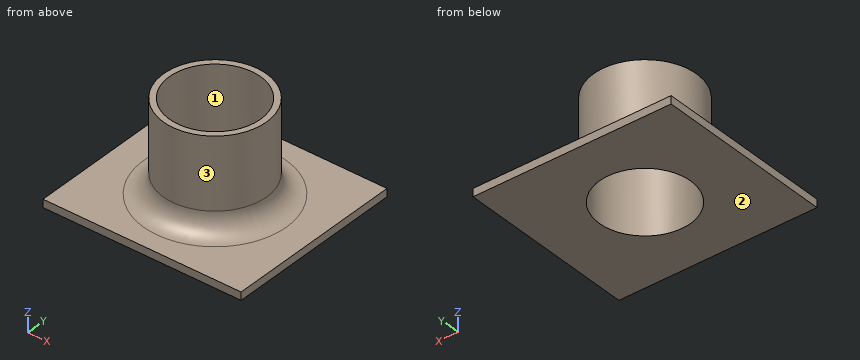
```python
from build123d import *

# Parameters (mm, degrees)
F1_W      = 50
F1_H      = 45.323998
F2_DEPTH  = 2
F0_R      = 13
F0_R_2    = 11.5
F3_DEPTH  = 25
F3_FACE_R = 11.5
F4_DEPTH  = 25
F5_R      = 5


with BuildPart() as f2:
    # F1 (on Top) → F2 (new body)
    with BuildSketch(Plane.XY):
        Rectangle(F1_W, F1_H)
    extrude(amount=F2_DEPTH)

    # F0 (on Top) → F3 (join)
    with BuildSketch(Plane.XY):
        Circle(F0_R)
        Circle(F0_R_2, mode=Mode.SUBTRACT)
    extrude(amount=F3_DEPTH)

    # F3_face (on face) → F4 (cut)
    with BuildSketch(Plane.XY.offset(2)):
        Circle(F3_FACE_R)
    extrude(amount=-F4_DEPTH, mode=Mode.SUBTRACT)

    # F5
    f5_edges = [f2.edges().sort_by_distance(p)[0] for p in [
        (-13, 0, 2),
    ]]
    fillet(f5_edges, radius=F5_R)


solid = f2.part
```
Can you work these out from the model? Positions are in its coordinate system, mm. Face numbers are marked on the shaded views. Round coordinates to 2 decimals unless told otherwise and drop trailing zeros. Loops run counter-clockwise (first coordinate to the right, second up) from the corner with the lowest first, then second, coordinate; pieces in that order, holes last. Notation, with made-up numbers: (0.25, -34.75) -> (34.25, -34.75) arc R8 cw to (34.25, -30.75) -> close; hole circle Ø2 at (0, 73). An arc over 180 degrees is marked (long way). Answer in a Markdown table with one row per item.
Item 1: If I drill on probe 1 along Y at (x, z) = (0, 10.25); probe 2 along Z at (x, y) = (-16, -13.5); probe 3 along X at (y, z) = (8, 12.25), over which ranges is the centre line in solid material (lowest first)?
Answer block:
| item | result |
|---|---|
| probe 1 | -13 to -11.5, 11.5 to 13 |
| probe 2 | 0 to 2 |
| probe 3 | -10.25 to -8.26, 8.26 to 10.25 |
Item 2: We'd pull the mould along X, two halves only. Please class the marked faces 1, 2 and 3: released by +X, released by -X, zero draft, split by the parting line, or undercut.
Answer block:
| item | result |
|---|---|
| face 1 | undercut |
| face 2 | zero draft |
| face 3 | split by the parting line |
Item 3: Will these pins go through, and if not, where does the flat tip stop? P1, Ø1, axis at y = -9.5, z = 10, coming from the +X side; P2, Ø1, axis at y = 6, z = 16, coming from the +X side; P3, Ø1.5, axis at y = -10, z = 10.5, coming from the -X side.
Answer block:
| item | result |
|---|---|
| P1 | x = 9.38 |
| P2 | x = 11.78 |
| P3 | x = -9.13 |
Item 4: Suppose I cut it at A-A, the plane y = 0. List the corners of the cut face in (x, z) for me.
Answer block:
| item | result |
|---|---|
| outline | (-25, 0) -> (-11.5, 0) -> (-11.5, 25) -> (-13, 25) -> (-13, 7) arc R5 cw to (-18, 2) -> (-25, 2) -> close; (11.5, 0) -> (25, 0) -> (25, 2) -> (18, 2) arc R5 cw to (13, 7) -> (13, 25) -> (11.5, 25) -> close |
Item 5: Suppose I cut it at B-B, the plane x = 0. List the corners of the cut face in (y, z) for me, plus the area to 3 significant figures.
Answer block:
| item | result |
|---|---|
| outline | (-22.66, 0) -> (-11.5, 0) -> (-11.5, 25) -> (-13, 25) -> (-13, 7) arc R5 cw to (-18, 2) -> (-22.66, 2) -> close; (11.5, 0) -> (22.66, 0) -> (22.66, 2) -> (18, 2) arc R5 cw to (13, 7) -> (13, 25) -> (11.5, 25) -> close |
| area | 124 mm² |
Item 6: Suppose I cut it at C-C, the plane z = 13.5. List the corners of the cut face in (x, y) for me, plus the area to 3 significant figures.
Answer block:
| item | result |
|---|---|
| outline | circle Ø26 at (0, 0); hole circle Ø23 at (0, 0) |
| area | 115 mm² |
